```python
from build123d import *

# Parameters (mm, degrees)
ESQUISSE1_W             = 40
ESQUISSE1_H             = 7
BOSS_EXTRU_1_DEPTH      = 8
ESQUISSE2_R             = 1.4
ENL_V_MAT_EXTRU_1_DEPTH = 42.388404173
ESQUISSE3_R             = 1.65
ENL_V_MAT_EXTRU_2_DEPTH = 42.388404173


with BuildPart() as part:
    # Esquisse1 → Boss.-Extru.1 (new body)
    with BuildSketch(Plane.XY):
        with Locations((20, 3.5)):
            Rectangle(ESQUISSE1_W, ESQUISSE1_H)
    extrude(amount=BOSS_EXTRU_1_DEPTH)

    # Esquisse2 → Enlèv. mat.-Extru.1 (cut, through all)
    with BuildSketch(Plane.XY.offset(8)):
        with Locations((20, 4.2)):
            Circle(ESQUISSE2_R)
        with Locations((3, 4.2)):
            Circle(ESQUISSE2_R)
        with Locations(Location((37, 4.2, 0), (0, 0, 180))):
            Circle(ESQUISSE2_R)
    extrude(amount=-ENL_V_MAT_EXTRU_1_DEPTH, mode=Mode.SUBTRACT)

    # Esquisse3 → Enlèv. mat.-Extru.2 (cut, through all)
    with BuildSketch(Plane(origin=(0, 7, 0), x_dir=(1, 0, 0), z_dir=(0, 1, 0))):
        with Locations(Location((8, -4, 0), (0, 0, 270))):
            Circle(ESQUISSE3_R)
        with Locations(Location((32, -4, 0), (0, 0, 90))):
            Circle(ESQUISSE3_R)
    extrude(amount=-ENL_V_MAT_EXTRU_2_DEPTH, mode=Mode.SUBTRACT)


solid = part.part
```
Design review of the part built by this model. Coordinates are the model's own, in mm. Round coordinates to 2 decimals unless told otherwise and drop trailing zeros. Write each loop counter-clockwise with the first axis right and the second up, starting at its lowest first coordinate (ties: lowest second). Pieces come first, ordered by that corner, then holes.
Item 1: We need section D-D on z = 1.75. Write out the cut boundary in (x, y), and give its area (3 significant figures).
Item 2: The part is to be moulded in two halves that separate along Y. For faces 1 (the flat face through (20, 7, 4)), 2 (the cylindrical face through (2.82, 5.59, 4.06)), 3 (the flat face through (20, 2, 8)), say which applies: +Y half, -Y half, draft (parallel to the pull), parting line (faces both ways), or undercut.
Item 3: For probe 1 along X at (y, z) = (4.25, 4); probe 2 along X at (y, z) = (4.5, 6.25); probe 3 along X at (y, z) = (2.75, 2.5), list the stretches that pass through material, from the lowest coordinate up.
Item 4: We need section B-B on z = 4. Write out the cut boundary in (x, y).
Item 5: We need section A-A on x = 20. Write out the cut boundary in (y, z).
Item 6: We need section C-C on y = 0.5. Write out the cut boundary in (x, z).
Returned:
1. outline: (0, 0) - (40, 0) - (40, 7) - (0, 7) - close; hole circle Ø2.8 at (3, 4.2); hole circle Ø2.8 at (20, 4.2); hole circle Ø2.8 at (37, 4.2)
1. area: 262 mm2
2. face 1: +Y half
2. face 2: undercut
2. face 3: draft
3. probe 1: x = 0 to 1.6, 4.4 to 6.35, 9.65 to 18.6, 21.4 to 30.35, 33.65 to 35.6, 38.4 to 40
3. probe 2: x = 0 to 1.63, 4.37 to 18.63, 21.37 to 35.63, 38.37 to 40
3. probe 3: x = 0 to 7.31, 8.69 to 31.31, 32.69 to 40
4. outline: (0, 0) - (6.35, 0) - (6.35, 7) - (0, 7) - close; (9.65, 0) - (30.35, 0) - (30.35, 7) - (9.65, 7) - close; (33.65, 0) - (40, 0) - (40, 7) - (33.65, 7) - close; hole circle Ø2.8 at (3, 4.2); hole circle Ø2.8 at (20, 4.2); hole circle Ø2.8 at (37, 4.2)
5. outline: (0, 0) - (2.8, 0) - (2.8, 8) - (0, 8) - close; (5.6, 0) - (7, 0) - (7, 8) - (5.6, 8) - close
6. outline: (0, 0) - (40, 0) - (40, 8) - (0, 8) - close; hole circle Ø3.3 at (8, 4); hole circle Ø3.3 at (32, 4)
